```python
from build123d import *

# Parameters (mm, degrees)
F1_DEPTH = 406.4
F2_R     = 12.7
F3_W     = 8
F3_H     = 22.225
F4_DEPTH = 26.924
F5_W     = 66.04
F5_H     = 33.02
F5_R     = 15.875
F6_DEPTH = 9.525


with BuildPart() as f1:
    # F0 (on Front) → F1 (new body)
    with BuildSketch(Plane.XZ):
        Polygon((-16, 0), (0, 0), (177.8, 0), (193.8, 0), (193.8, 4), (177.8, 4), (177.8, 165.1), (0, 165.1), (0, 4), (-16, 4), align=None)
    extrude(amount=F1_DEPTH)

    # F2
    f2_edges = [f1.edges().sort_by_distance(p)[0] for p in [
        (193.8, 0, 2),
        (193.8, -406.4, 2),
        (-16, -406.4, 2),
        (-16, 0, 2),
    ]]
    fillet(f2_edges, radius=F2_R)

    # F3 (on face) → F4 (join)
    with BuildSketch(Plane.XZ.offset(406.4)):
        with Locations((69.532, 36.5125)):
            Rectangle(F3_W, F3_H)
        with Locations((105.6, 22.2885)):
            Rectangle(F3_W, F3_H)
    extrude(amount=F4_DEPTH)

    # F5 (on face) → F6 (join)
    with BuildSketch(Plane(origin=(0, 0, 0), x_dir=(-1, 0, 0), z_dir=(0, 1, 0))):
        with Locations((-62.865, 44.45)):
            Rectangle(F5_W, F5_H)
        with Locations((-127, 44.45)):
            Circle(F5_R)
    extrude(amount=F6_DEPTH)


solid = f1.part
```
Can you work these out from the model? Positions are in its coordinate system, mm. A direction names the side the tool comes from. Coordinates: 2 decimals unless noted, no trailing zeros. Write each loop counter-clockwise with the first axis right and the second up, starting at its lowest first coordinate (ties: lowest second). Pieces come first, ordered by that corner, then holes. Notation, with made-up numbers: (67.25, -7.5) - (97.25, -7.5) arc R20 cw to (97.25, -2.5) - close; hole circle Ø3 at (60.25, -24). An arc over 180 degrees is marked (long way). Return JSON: item names as keys, results as strings.
Q1. I'm going to push flat-ended pins straight in: pin 1 Ø5 at (x, y) = (-11, -227) entering from +Z; pin 2 Ø1.5 at (x, z) = (96, 62.5) entering from -Y; pin 3 Ø3 at (y, z) = (3, 42) entering from -X (3 decimals). Where does each tip first touch, or does it pass through?
Computed values:
{"pin 1": "stops at z = 4", "pin 2": "stops at y = -406.4", "pin 3": "stops at x = 29.845"}
Q2. Please list where these lines run through material, in increasing order: L1, parallel to Y at x = 132.5, z = 143.5; L2, parallel to X at y = -384, z = 85.5; L3, parallel to Z at x = -5.5, y = -336. Write a range as from..to.
Computed values:
{"L1": "y = -406.4..0", "L2": "x = 0..177.8", "L3": "z = 0..4"}
Q3. If we section it at C-C (z = 143): Please give me the cut outline in (x, y), then the cut area to 3 significant figures.
Computed values:
{"outline": "(0, -406.4) - (177.8, -406.4) - (177.8, 0) - (0, 0) - close", "area": "72,300 mm2"}
Q4. On a 3-axis mill with a long thin cutter (end or side, diameter ignored), from which of +Z, -Z, +X, -X, +Y, -Y can I reach the whole of each face in a straight line? I mean faces 1 (the flat face through (106, -420, 11.176)), 2 (the flat face through (-8, -200, 4)), 3 (the flat face through (109.6, -420, 22)), 4 (the flat face through (177.8, -200, 83)). Say none if no direction works.
Computed values:
{"face 1": "-Z, +X, -X, -Y", "face 2": "+Z, -X, +Y, -Y", "face 3": "+Z, -Z, +X, -Y", "face 4": "+Z, +X, +Y, -Y"}
Q5. Thinking about a two-plate mould opening in X: for faces 5 (the flat face through (29.845, 5, 44)), 6 (the flat face through (106, -420, 33.401)), 7 (the flat face through (95.885, 5, 44)), which applies, +X half, -X half, draft (parallel to the pull), parting line (faces both ways), or undercut?
Computed values:
{"face 5": "-X half", "face 6": "draft", "face 7": "undercut"}
Q6. If we section it at A-A (y = -168.5): Please give me the cut outline in (x, z).
Computed values:
{"outline": "(-16, 0) - (193.8, 0) - (193.8, 4) - (177.8, 4) - (177.8, 165.1) - (0, 165.1) - (0, 4) - (-16, 4) - close"}
Q7. If we section it at B-B (x = 89): Please give me the cut outline in (y, z) (3 decimals), then the cut area to 3 significant figures.
Computed values:
{"outline": "(-406.4, 0) - (0, 0) - (0, 27.94) - (9.525, 27.94) - (9.525, 60.96) - (0, 60.96) - (0, 165.1) - (-406.4, 165.1) - close", "area": "67,400 mm2"}
